from build123d import *

# Parameters (mm, degrees)
SKETCH1_R           = 1.5
BOSS_EXTRUDE1_DEPTH = 3
SKETCH2_W           = 51
SKETCH2_H           = 40.3
BOSS_EXTRUDE2_DEPTH = 3
SKETCH3_W           = 33
SKETCH3_H           = 40.3
SKETCH3_R           = 1.4
BOSS_EXTRUDE3_DEPTH = 3
SKETCH5_W           = 27
SKETCH5_H           = 40.3
SKETCH5_R           = 1.4
BOSS_EXTRUDE4_DEPTH = 3


with BuildPart() as part:
    # Sketch1 → Boss-Extrude1 (new body)
    with BuildSketch(Plane.XY):
        Polygon((-28.851027023, -20.15), (-28.851027023, -13), (-28.851027023, -6.5), (-36.501027023, -6.5), (-36.501027023, -16.735786438), (-33.086813461, -20.15), align=None)
        with Locations((-31.851027023, -15.5)):
            Circle(SKETCH1_R, mode=Mode.SUBTRACT)
        Polygon((-36.501027023, 16.735786438), (-36.501027023, 6.5), (-28.851027023, 6.5), (-28.851027023, 20.15), (-33.086813461, 20.15), align=None)
        with Locations((-31.851027023, 15.5)):
            Circle(SKETCH1_R, mode=Mode.SUBTRACT)
        Polygon((-36.501027023, -20.15), (-33.086813461, -20.15), (-36.501027023, -16.735786438), align=None)
        Polygon((-36.501027023, 20.15), (-36.501027023, 16.735786438), (-33.086813461, 20.15), align=None)
        Polygon((-36.501027023, -16.735786438), (-36.501027023, -6.5), (-36.501027023, 6.5), (-36.501027023, 16.735786438), (-36.501027023, 20.15), (-41.501027023, 20.15), (-41.501027023, -20.15), (-36.501027023, -20.15), align=None)
    extrude(amount=BOSS_EXTRUDE1_DEPTH)

    # Sketch2 → Boss-Extrude2 (add)
    with BuildSketch(Plane(origin=(-41.501027023, 0, 0), x_dir=(0, 0, -1), z_dir=(1, 0, 0))):
        with Locations((25.5, 0)):
            Rectangle(SKETCH2_W, SKETCH2_H)
    extrude(amount=BOSS_EXTRUDE2_DEPTH)

    # Sketch3 → Boss-Extrude3 (add)
    with BuildSketch(Plane(origin=(0, 0, -51), x_dir=(-1, 0, 0), z_dir=(0, 0, -1))):
        with Locations((25.001027023, 0)):
            Rectangle(SKETCH3_W, SKETCH3_H)
        with Locations((30.251027023, 5.15)):
            Circle(SKETCH3_R, mode=Mode.SUBTRACT)
        with Locations((30.251027023, -4.85)):
            Circle(SKETCH3_R, mode=Mode.SUBTRACT)
    extrude(amount=BOSS_EXTRUDE3_DEPTH)

    # Sketch5 → Boss-Extrude4 (add)
    with BuildSketch(Plane(origin=(-8.501027023, 0, 0), x_dir=(0, 0, -1), z_dir=(1, 0, 0))):
        with Locations((64.5, 0)):
            Rectangle(SKETCH5_W, SKETCH5_H)
        with Locations((71, 0)):
            Circle(SKETCH5_R, mode=Mode.SUBTRACT)
        with Locations((61, 0)):
            Circle(SKETCH5_R, mode=Mode.SUBTRACT)
    extrude(amount=BOSS_EXTRUDE4_DEPTH)


solid = part.part
Part model, mm, in its own coordinate system. A direction names the side the tool comes from. Give positions to 0.01 mm unless a question says otherwise; leave off trailing zeros. Loops run counter-clockwise (first coordinate to the right, second up) from the corner with the lowest first, then second, coordinate; pieces in that order, holes last. Notation, with made-up numbers: M 60.25,-13.5 L 118.25,-13.5 A33 ccw 118.25,17.5 Z; hole C 62,60.25 d6. An arc over 180 degrees is marked long. Put each result on its own line as item: value. Start each with the question number.
1) 3-axis set-ups, long thin cutter, end or side, ignore diameter. For faces 5 (the flat face through (-37, 0, 0)), 6 (the flat face through (-8.501, 0, -66)), 7 (the flat face through (-33, 6.5, 1)): which of +Z, -Z, +X, -X, +Y, -Y reach the whole face in a straight line?
2) Saw through at A-A (y = 5.15). List the corners of the cut face in (x, z), then the cut area to 3 significant figures.
3) Flat gauge pins, fed straight in: pin 1 (0.9 mm diameter, centred on y = -10.5, z = 2, fed in from +X); pin 2 (1.5 mm diameter, centred on y = 1, z = -24, fed in from +X); pin 3 (5 mm diameter, centred on x = -36, y = -0.5, fed in from -Z). Where does each tip first touch, or does it go through?
4) Saw through at C-C (z = -71). List the corners of the cut face in (x, y).
5) Saw through at D-D (y = -15.5). List the corners of the cut face in (x, z).
6) Saw through at B-B (x = -37.5). List the corners of the cut face in (y, z).
7) Probe probe 1 along Z at (x, y) = (-36.5, -9); probe 2 along Y at (x, z) = (-6.6, -61); probe 3 along X at (y, z) = (-3, -24.5). List the from-to ranges inside material, lowest first.
8) Pull direction X, two halves, no side cores. Call faces 1 (the cylindrical face through (-28.852, 5.212, -52.479)), 2 (the cylindrical face through (-30.42, -15.05, 1.48)), 3 (the flat face through (-41.501, 0, -25)), 4 (the flat face through (-37, 0, 3)): +X half, -X half, draft (parallel to the pull), parting line (faces both ways), or undercut.
Numbers:
1. face 5: +X, +Y, -Y
1. face 6: -Z, -X, +Y, -Y
1. face 7: +Z, +X
2. outline: M -41.5,-54 L -31.65,-54 L -31.65,-51 L -38.5,-51 L -38.5,0 L -36.5,0 L -36.5,3 L -41.5,3 Z; M -28.85,-54 L -8.5,-54 L -8.5,-78 L -5.5,-78 L -5.5,-51 L -28.85,-51 Z
2. area: 340 mm^2
3. pin 1: x = -28.85
3. pin 2: x = -38.5
3. pin 3: z = -54
4. outline: M -8.5,-20.15 L -5.5,-20.15 L -5.5,-1.4 L -8.5,-1.4 Z; M -8.5,1.4 L -5.5,1.4 L -5.5,20.15 L -8.5,20.15 Z
5. outline: M -41.5,-54 L -8.5,-54 L -8.5,-78 L -5.5,-78 L -5.5,-51 L -38.5,-51 L -38.5,0 L -33.35,0 L -33.35,3 L -41.5,3 Z; M -30.35,0 L -28.85,0 L -28.85,3 L -30.35,3 Z
6. outline: M -20.15,-54 L 20.15,-54 L 20.15,-51 L -20.15,-51 Z; M -20.15,0 L 20.15,0 L 20.15,3 L -20.15,3 Z
7. probe 1: -54 to -51, 0 to 3
7. probe 2: -20.15 to -1.4, 1.4 to 20.15
7. probe 3: -41.5 to -38.5
8. face 1: undercut
8. face 2: undercut
8. face 3: -X half
8. face 4: draft
